Design review of the part built by this model. Coordinates are the model's own, in mm. A direction names the side the tool comes from. Give positions to 0.01 mm unless a question says otherwise; leave off trailing zeros. Write each loop counter-clockwise with the first axis right and the second up, starting at its lowest first coordinate (ties: lowest second). Pieces come first, ordered by that corner, then holes.
```python
from build123d import *

# Parameters (mm, degrees)
SKETCH1_W               = 76.2
SKETCH1_H               = 304.8
BOSS_EXTRUDE1_DEPTH     = 1.5875
SKETCH2_R               = 6.35
BOSS_EXTRUDE2_DEPTH     = 304.8
CUT_EXTRUDE1_REACH      = 310.693
SKETCH5_R               = 5.020069527
CUT_EXTRUDE2_DEPTH      = 22.4155
CUT_EXTRUDE2_DEPTH_BACK = 22.4155
SKETCH6_W               = 31.253930699
SKETCH6_H               = 25.4
SKETCH6_W_2             = 35.598147882
SKETCH6_W_3             = 29.083231171


with BuildPart() as part:
    # Sketch1 → Boss-Extrude1 (new body)
    with BuildSketch(Plane.XY):
        with Locations((-2.744516439, 43.403238015)):
            Rectangle(SKETCH1_W, SKETCH1_H)
    extrude(amount=BOSS_EXTRUDE1_DEPTH)

    # Sketch2 → Boss-Extrude2 (add)
    with BuildSketch(Plane(origin=(0, 195.803238015, 0), x_dir=(1, 0, 0), z_dir=(0, 1, 0))):
        with Locations((-40.844516439, -6.35)):
            Circle(SKETCH2_R)
    extrude(amount=-BOSS_EXTRUDE2_DEPTH)

    # Sketch5 → Cut-Extrude1 (cut, up to next)
    with BuildSketch(Plane(origin=(0, 195.803238015, 0), x_dir=(1, 0, 0), z_dir=(0, 1, 0)), mode=Mode.PRIVATE) as cut_extrude1_sk1:
        with Locations(Location((-40.844516439, -6.35, 0), (0, 0, 270))):
            Circle(SKETCH5_R)
    cut_extrude1_tool1 = extrude(cut_extrude1_sk1.sketch, amount=-CUT_EXTRUDE1_REACH, mode=Mode.PRIVATE) & part.part
    add(cut_extrude1_tool1.solids().sort_by_distance((-40.844516, 195.803238, 6.35))[0], mode=Mode.SUBTRACT)

    # Sketch6 → Cut-Extrude2 (cut, two sides: drawn at the far end of the back side and taken through both)
    with BuildSketch(Plane.XY.offset(1.5875).offset(-CUT_EXTRUDE2_DEPTH_BACK)):
        with Locations((-50.121481789, 183.103238015)):
            Rectangle(SKETCH6_W, SKETCH6_H)
        with Locations((-50.121481789, 132.303238015)):
            Rectangle(SKETCH6_W, SKETCH6_H)
        with Locations((-50.121481789, 81.503238015)):
            Rectangle(SKETCH6_W, SKETCH6_H)
        with Locations((-50.121481789, 30.703238015)):
            Rectangle(SKETCH6_W, SKETCH6_H)
        with Locations((-52.29359038, -20.096761985)):
            Rectangle(SKETCH6_W_2, SKETCH6_H)
        with Locations((-49.036132025, -70.896761985)):
            Rectangle(SKETCH6_W_3, SKETCH6_H)
    extrude(amount=CUT_EXTRUDE2_DEPTH + CUT_EXTRUDE2_DEPTH_BACK, mode=Mode.SUBTRACT)


solid = part.part
```
(1) To check wall thickness, follow L1, parallel to X at y = -47, z = 6.35; L2, parallel to Z at x = -1, y = 103; L3, parallel to Z at x = -42.5, y = -51. State the ranges of each line that lie inside material, in increasing order.
Resolved:
L1: x = -47.19 to -45.86, -35.82 to -34.49
L2: z = 0 to 1.59
L3: z = 0.22 to 1.61, 11.09 to 12.48
(2) Clearance check with flat-ended pins moving along their axes: P1, Ø2, axis at x = 13.5, z = 4.5, coming from the -Y side; P2, Ø1.7, axis at y = 86.5, z = 0.5, coming from the -X side; P3, Ø1, axis at x = -4.5, y = 106.5, coming from the +Z side. State where each tip first meets the part, or that it passes through.
Resolved:
P1: passes through
P2: stops at x = -34.49
P3: stops at z = 1.59
(3) Mouldability with a two-part tool opening along Y and no side actions: class faces 3 (the face through (-36, 170.403, 4)), 4 (the face through (-36, 119.603, 4)), 5 (the face through (-43.899, 107.081, 2.366)), 6 (the face through (-36, 145.003, 4)) as pulls with the +Y half, pulls with the -Y half, needs draft (parallel to the pull), parting line crosses it, or undercut.
Resolved:
face 3: pulls with the +Y half
face 4: undercut
face 5: needs draft
face 6: undercut
(4) Consider section C-C, the plane x = 0.5. Give the boundary of the cut face in (y, z).
Resolved:
outline: (-109, 0) - (195.8, 0) - (195.8, 1.59) - (-109, 1.59) - close
(5) Tool access review of faces 1 (the face through (-43.899, -45.319, 2.366)), 2 (the face through (-36, -58.197, 4)): name each direction out of +Z, -Z, +X, -X, +Y, -Y from which nothing blocks a thin tool from reaching the whole face with its end or side.
Resolved:
face 1: +Y, -Y
face 2: +Z, -Z, -X
(6) Consider section B-B, the plane y = 37. Give the boundary of the cut face in (x, z), then the cut area to 3 significant figures.
Resolved:
outline: (-34.49, 0) - (35.36, 0) - (35.36, 1.59) - (-34.49, 1.59) - close
area: 111 mm2
(7) Consider section A-A, the plane z = 6.35. Give the number of separate pieces and of enclosed holes in the cut face, then the cut area to 3 significant figures.
Resolved:
separate pieces: 12
enclosed holes: 0
area: 405 mm2
